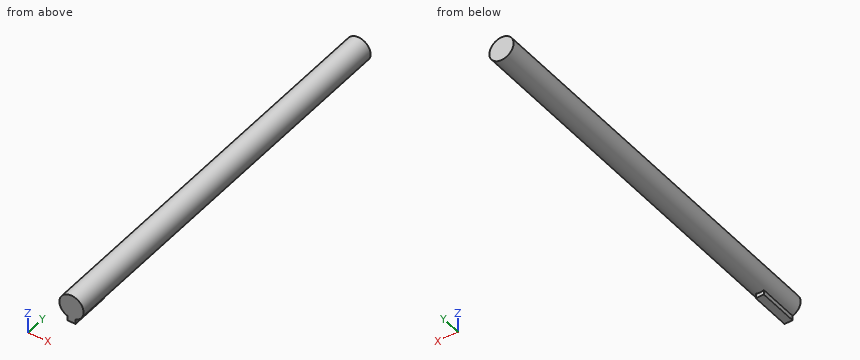
```python
from build123d import *

# Parameters (mm, degrees)
SKETCH_1_R      = 3
EXTRUDE_1_DEPTH = 100
SKETCH_2_W      = 2
SKETCH_2_H      = 2
EXTRUDE_2_DEPTH = 10


with BuildPart() as part:
    # 스케치1 → 보스-돌출1 (new body)
    with BuildSketch(Plane(origin=(0, 0, 0), x_dir=(1, 0, 0), z_dir=(0, 1, 0))):
        with Locations(Location((0, 0, 0), (0, 0, 270))):
            Circle(SKETCH_1_R)
    extrude(amount=EXTRUDE_1_DEPTH)

    # 스케치2 → 보스-돌출2 (add)
    with BuildSketch(Plane(origin=(0, 0, 0), x_dir=(1, 0, 0), z_dir=(0, 1, 0))):
        with Locations((0, 3)):
            Rectangle(SKETCH_2_W, SKETCH_2_H)
    extrude(amount=EXTRUDE_2_DEPTH)


solid = part.part
```
CAD build for the part. Positions are in the model's coordinates, mm. Round coordinates to 2 decimals unless told otherwise and drop trailing zeros. Order: outer loops, then holes, each group sorted by start corner. A loop starts at its lowest first (then second) coordinate and runs counter-clockwise, first axis right, second up.
Item 1: Probe line 1 along Z through (x, y) = (0.35, 86.5); line 2 along Y through (x, z) = (0.3, -3.5); line 3 along X through (y, z) = (30, -0.5). List the from-to ranges inside material, lowest first.
Item 2: Pin check, flat tips, straight feed: pin 1 (2 mm diameter, centred on x = 0.5, y = 71.5, fed in from +Z); pin 2 (0.6 mm diameter, centred on y = 7.5, z = -3.5, fed in from -X); pin 3 (0.9 mm diameter, centred on x = 0.5, z = -3.5, fed in from +Y); pin 4 (1.5 mm diameter, centred on x = -2, y = 14.5, fed in from +Z). Stop position of each tip, or through.
Item 3: Saw through at C-C on y = 7. Write the cut outline in (x, z), then the cut area to 3 significant figures.
Item 4: Saw through at B-B on y = 63. Write the cut outline in (x, z).
Item 5: Saw through at D-D on z = 2. Write the cut outline in (x, y), then the cut area to 3 significant figures.
Item 6: Saw through at A-A on x = 0. Write the cut outline in (y, z), then the cut area to 3 significant figures.
Reported:
1. line 1: z = -2.98 to 2.98
1. line 2: y = 0 to 10
1. line 3: x = -2.96 to 2.96
2. pin 1: stops at z = 3
2. pin 2: stops at x = -1
2. pin 3: stops at y = 10
2. pin 4: stops at z = 2.73
3. outline: (-1, -4) - (1, -4) - (1, -2.83) arc R3 ccw (long way) to (-1, -2.83) - close
3. area: 30.4 mm2
4. outline: circle Ø6 at (0, 0)
5. outline: (-2.24, 0) - (2.24, 0) - (2.24, 100) - (-2.24, 100) - close
5. area: 447 mm2
6. outline: (0, -4) - (10, -4) - (10, -3) - (100, -3) - (100, 3) - (0, 3) - close
6. area: 610 mm2
